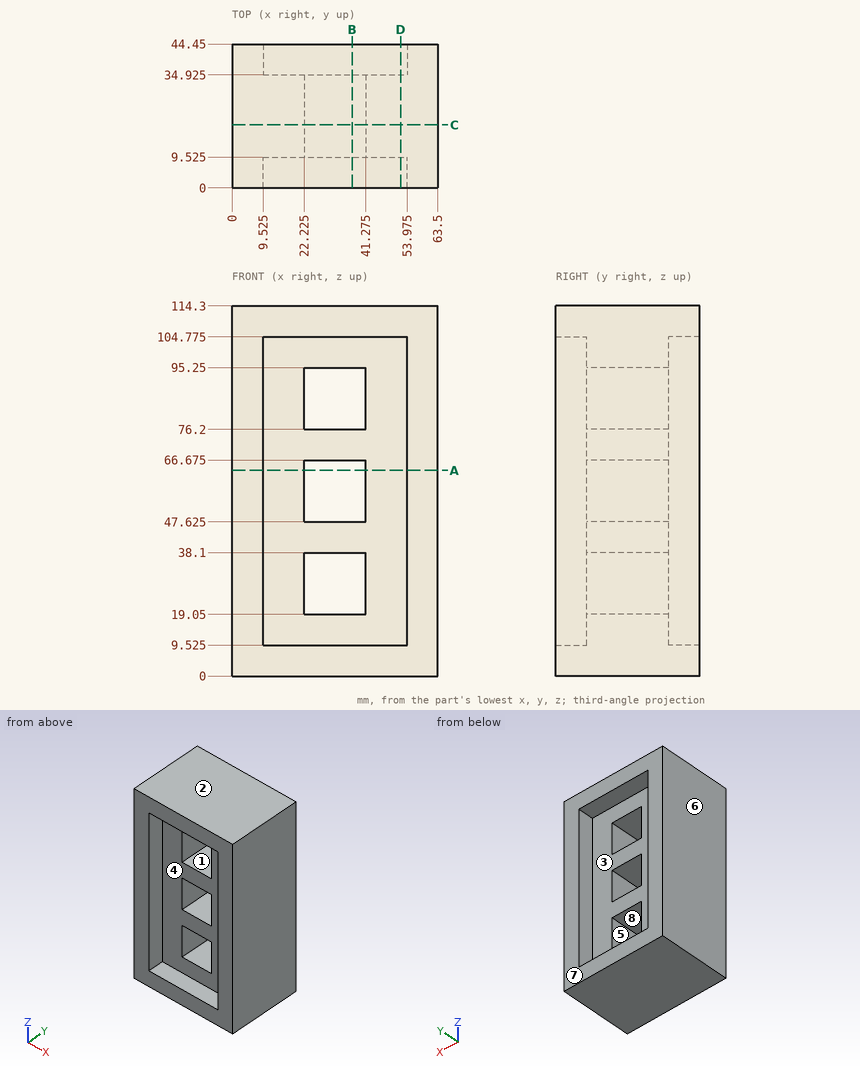
Geometry check sheet. Reference: drawing and pictorial views, mm from the part's lowest x, y, z. A direction names the side the tool comes from. Round coordinates to 2 decimals unless told otherwise and drop trailing zeros. Order: outer loops, then holes, each group sorted by start corner. A loop starts at its lowest first (then second) coordinate and runs counter-clockwise, first axis right, second up.
Q1. Set-up check for the marked faces 1, 2, 3 and 4: record each of +Z, -Z, +X, -X, +Y, -Y from which the full face is reachable in a straight line by a thin tool's end or side.
Filled sheet:
face 1: +Y, -Y
face 2: +Z, +X, -X, +Y, -Y
face 3: +Y
face 4: -Y
Q2. Scan lines: L1, parallel to Z at x = 37, y = 16 (3 decimals); L2, parallel to Z at x = 39.5, y = 7 (3 decimals); L3, parallel to X at y = 21, z = 31.5 (3 decimals). Record each from-to range of solid material in increasing order.
Filled sheet:
L1: z = 0 to 19.05, 38.1 to 47.625, 66.675 to 76.2, 95.25 to 114.3
L2: z = 0 to 9.525, 104.775 to 114.3
L3: x = 0 to 22.225, 41.275 to 63.5
Q3. Depth check by flat-ended pin: P1, Ø1, axis at x = 51, z = 64.5, coming from the +Y side (3 decimals); P2, Ø22, axis at x = 28.5, z = 42.5, coming from the -Y side (3 decimals). Enter the tip coordinate at first touch or a pass-through.
Filled sheet:
P1: stops at y = 34.925
P2: stops at y = 9.525
Q4. Cross-section at C-C, the plane y = 19.5. Enter the section's corners in (x, z) (3 decimals).
Filled sheet:
outline: (0, 0) - (63.5, 0) - (63.5, 114.3) - (0, 114.3) - close; hole (22.225, 19.05) - (41.275, 19.05) - (41.275, 38.1) - (22.225, 38.1) - close; hole (22.225, 47.625) - (41.275, 47.625) - (41.275, 66.675) - (22.225, 66.675) - close; hole (22.225, 76.2) - (41.275, 76.2) - (41.275, 95.25) - (22.225, 95.25) - close
Q5. Cross-section at B-B, the plane x = 37. Enter the section's corners in (y, z) (3 decimals).
Filled sheet:
outline: (0, 0) - (44.45, 0) - (44.45, 9.525) - (34.925, 9.525) - (34.925, 19.05) - (9.525, 19.05) - (9.525, 9.525) - (0, 9.525) - close; (0, 104.775) - (9.525, 104.775) - (9.525, 95.25) - (34.925, 95.25) - (34.925, 104.775) - (44.45, 104.775) - (44.45, 114.3) - (0, 114.3) - close; (9.525, 38.1) - (34.925, 38.1) - (34.925, 47.625) - (9.525, 47.625) - close; (9.525, 66.675) - (34.925, 66.675) - (34.925, 76.2) - (9.525, 76.2) - close
Q6. Cross-section at D-D, the plane x = 52. Enter the section's corners in (y, z) (3 decimals).
Filled sheet:
outline: (0, 0) - (44.45, 0) - (44.45, 9.525) - (34.925, 9.525) - (34.925, 104.775) - (44.45, 104.775) - (44.45, 114.3) - (0, 114.3) - (0, 104.775) - (9.525, 104.775) - (9.525, 9.525) - (0, 9.525) - close
Q7. Draft check along X on the marked faces 5, 6, 7 and 8. Enter one of: pulls with the +X half, pulls with the -X half, needs draft (parallel to the pull), parting line crosses it, or undercut.
Filled sheet:
face 5: undercut
face 6: pulls with the -X half
face 7: needs draft
face 8: undercut
Q8. Cross-section at A-A, the plane z = 63.5. Enter the section's corners in (x, y) (3 decimals), plus the area to 3 significant figures.
Filled sheet:
outline: (0, 0) - (9.525, 0) - (9.525, 9.525) - (22.225, 9.525) - (22.225, 34.925) - (9.525, 34.925) - (9.525, 44.45) - (0, 44.45) - close; (41.275, 9.525) - (53.975, 9.525) - (53.975, 0) - (63.5, 0) - (63.5, 44.45) - (53.975, 44.45) - (53.975, 34.925) - (41.275, 34.925) - close
area: 1,490 mm2
